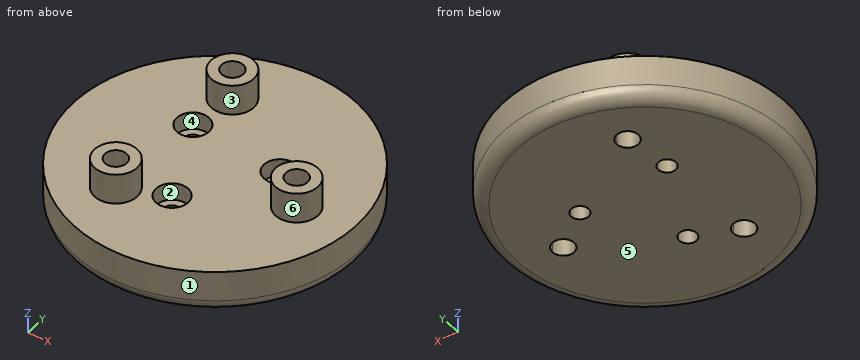
```python
from build123d import *

# Parameters (mm, degrees)
SKETCH1_R               = 16.25
SKETCH1_R_2             = 1
SKETCH1_R_3             = 1.25
BOSS_EXTRUDE1_DEPTH     = 5
FILLET1_R               = 1.5
SKETCH2_R               = 2.45
BOSS_EXTRUDE2_DEPTH     = 3.5
SKETCH4_R               = 1.25
CUT_EXTRUDE1_DEPTH      = 1
CUT_EXTRUDE1_DEPTH_BACK = 9.5
SKETCH5_R               = 1.85
CUT_EXTRUDE2_DEPTH      = 2


with BuildPart() as part:
    # Sketch1 → Boss-Extrude1 (new body)
    with BuildSketch(Plane.XY):
        Circle(SKETCH1_R)
        with Locations((-0.544723392, -6.226216863)):
            Circle(SKETCH1_R_2, mode=Mode.SUBTRACT)
        with Locations((-5.119700277, 3.584852727)):
            Circle(SKETCH1_R_2, mode=Mode.SUBTRACT)
        with Locations((5.664423669, 2.641364136)):
            Circle(SKETCH1_R_2, mode=Mode.SUBTRACT)
        with Locations((-5.591929035, -8.290375726)):
            Circle(SKETCH1_R_3, mode=Mode.SUBTRACT)
        with Locations((-4.383711468, 8.987940463)):
            Circle(SKETCH1_R_3, mode=Mode.SUBTRACT)
        with Locations((9.975640503, -0.697564737)):
            Circle(SKETCH1_R_3, mode=Mode.SUBTRACT)
    extrude(amount=BOSS_EXTRUDE1_DEPTH)

    # Fillet1
    fillet1_edges = [part.edges().sort_by_distance(p)[0] for p in [
        (-16.25, 0, 0),
    ]]
    fillet(fillet1_edges, radius=FILLET1_R)

    # Sketch2 → Boss-Extrude2 (add)
    with BuildSketch(Plane.XY.offset(5)):
        with Locations((-5.591929035, -8.290375726)):
            Circle(SKETCH2_R)
        with Locations((-4.383711468, 8.987940463)):
            Circle(SKETCH2_R)
        with Locations((9.975640503, -0.697564737)):
            Circle(SKETCH2_R)
    extrude(amount=BOSS_EXTRUDE2_DEPTH)

    # Sketch4 → Cut-Extrude1 (cut, two sides)
    with BuildSketch(Plane(origin=(0, 0, 0), x_dir=(-1, 0, 0), z_dir=(0, 0, -1))) as cut_extrude1_sk:
        with Locations((4.383711468, 8.987940463)):
            Circle(SKETCH4_R)
        with Locations((-9.975640503, -0.697564737)):
            Circle(SKETCH4_R)
        with Locations((5.591929035, -8.290375726)):
            Circle(SKETCH4_R)
    extrude(amount=CUT_EXTRUDE1_DEPTH, mode=Mode.SUBTRACT)
    extrude(cut_extrude1_sk.sketch, amount=-CUT_EXTRUDE1_DEPTH_BACK, mode=Mode.SUBTRACT)

    # Sketch5 → Cut-Extrude2 (cut)
    with BuildSketch(Plane.XY.offset(5)):
        with Locations((5.664423669, 2.641364136)):
            Circle(SKETCH5_R)
        with Locations((-5.119700277, 3.584852727)):
            Circle(SKETCH5_R)
        with Locations((-0.544723392, -6.226216863)):
            Circle(SKETCH5_R)
    extrude(amount=-CUT_EXTRUDE2_DEPTH, mode=Mode.SUBTRACT)


solid = part.part
```
Build history of the part. All positions in model axes, mm. Face numbers are marked on the shaded views. A direction names the side the tool comes from. Give positions to 0.01 mm unless a question says otherwise; leave off trailing zeros. Loops run counter-clockwise (first coordinate to the right, second up) from the corner with the lowest first, then second, coordinate; pieces in that order, holes last. Notation, with made-up numbers: (-22.75, 22) - (25.25, 22) arc R34 cw to (25.25, 53) - close; hole circle Ø6 at (28, 58). An arc over 180 degrees is marked (long way). Use a Markdown table: item, result.
(1) Wall check: line 1 along X through (y, z) = (9, 6.25); line 2 along Z through (x, y) = (14, 1.5); line 3 along Z through (x, y) = (5, 1). Give the ranges that are in metal, low to high.
Taken from the geometry:
| item | result |
|---|---|
| line 1 | -6.83 to -5.63, -3.13 to -1.93 |
| line 2 | 0 to 5 |
| line 3 | 0 to 3 |
(2) Which spindle directions (+Z, -Z, +X, -X, +Y, -Y) get a long thin tool onto all of the face, cutting with end or side? Do the marked faces 1 and 2. Say none if no direction does.
Taken from the geometry:
| item | result |
|---|---|
| face 1 | +Z, -Z |
| face 2 | +Z |
(3) Band-saw the part on C-C (x = 0). Give the cut face in (y, z).
Taken from the geometry:
| item | result |
|---|---|
| outline | (-16.25, 1.5) arc R1.5 ccw to (-14.75, 0) - (-7.06, 0) - (-7.06, 3) - (-7.99, 3) - (-7.99, 5) - (-16.25, 5) - close; (-5.39, 0) - (14.75, 0) arc R1.5 ccw to (16.25, 1.5) - (16.25, 5) - (-4.46, 5) - (-4.46, 3) - (-5.39, 3) - close |
(4) Pull direction Y, two halves, no side cores. Call the marked faces 3, 4, 5 and 6: +Y half, -Y half, draft (parallel to the pull), parting line (faces both ways), or undercut.
Taken from the geometry:
| item | result |
|---|---|
| face 3 | undercut |
| face 4 | undercut |
| face 5 | draft |
| face 6 | parting line |
(5) Band-saw the part on A-A (z = 5.5). Give the cut face in (x, y).
Taken from the geometry:
| item | result |
|---|---|
| outline | circle Ø4.9 at (-5.59, -8.29); circle Ø4.9 at (-4.38, 8.99); circle Ø4.9 at (9.98, -0.7); hole circle Ø2.5 at (-5.59, -8.29); hole circle Ø2.5 at (-4.38, 8.99); hole circle Ø2.5 at (9.98, -0.7) |
(6) Band-saw the part on B-B (y = 0). Give the cut face in (x, z).
Taken from the geometry:
| item | result |
|---|---|
| outline | (-16.25, 1.5) arc R1.5 ccw to (-14.75, 0) - (8.94, 0) - (8.94, 8.5) - (7.63, 8.5) - (7.63, 5) - (-16.25, 5) - close; (11.01, 0) - (14.75, 0) arc R1.5 ccw to (16.25, 1.5) - (16.25, 5) - (12.32, 5) - (12.32, 8.5) - (11.01, 8.5) - close |
(7) Band-saw the part on D-D (z = 2.25). Give the cut face in (x, y).
Taken from the geometry:
| item | result |
|---|---|
| outline | circle Ø32.5 at (0, 0); hole circle Ø2.5 at (-5.59, -8.29); hole circle Ø2 at (-5.12, 3.58); hole circle Ø2.5 at (-4.38, 8.99); hole circle Ø2 at (-0.54, -6.23); hole circle Ø2 at (5.66, 2.64); hole circle Ø2.5 at (9.98, -0.7) |
(8) Drop flat-ended pins along their axis: pin 1 Ø1.8 at (x, y) = (-5, 4) entering from +Z; pin 2 Ø6 at (x, y) = (5.66, 2.64) entering from -Z; pin 3 Ø1.5 at (x, y) = (-12, 3.5) entering from +Z; pin 4 Ø1.5 at (x, y) = (-5.59, -8.29) entering from -Z. Give the stop position or say it passes through.
Taken from the geometry:
| item | result |
|---|---|
| pin 1 | z = 3 |
| pin 2 | z = 0 |
| pin 3 | z = 5 |
| pin 4 | through |
